The model under review builds one solid part; all positions refer to its coordinate system, in mm. Face numbers are marked on the shaded views. A direction names the side the tool comes from. Give positions to 0.01 mm unless a question says otherwise; leave off trailing zeros. Order: outer loops, then holes, each group sorted by start corner. A loop starts at its lowest first (then second) coordinate and runs counter-clockwise, first axis right, second up. Notation, with made-up numbers: (-5, 64) - (13, 64) arc R18 ccw to (13, 89) - close; hole circle Ø8 at (17.25, 0.5). An arc over 180 degrees is marked (long way). Write item = value, one per line. Start each with the question number.
1. We need section A-A, the plane y = 11. Give the boundary of the cut face in (x, z) (3 decimals).
2. We need section D-D, the plane z = 30. Give the boundary of the cut face in (x, y) (3 decimals), and give its area (3 significant figures).
3. We need section B-B, the plane z = 16.5. Give the boundary of the cut face in (x, y), and give its area (3 significant figures).
4. Wall thickness on probe 1 along X at (y, z) = (7.75, 17.5) (3 decimals); probe 2 along Y at (x, z) = (-45.5, 17); probe 3 along Y at (x, z) = (-27, 2): over which ranges is each line inside the solid? List them lowest first.
5. For P1, Ø4, axis at y = -7, z = 26, coming from the +X side; P2, Ø4.5, axis at y = 1, z = 32.5, coming from the -X side; P3, Ø5.5, axis at y = 0, z = 30, coming from the -X side; P4, Ø3, axis at x = -7, y = 0, coming from the +Z side, all flat-tipped, find the tip position at first contact; note any pin that passes through.
6. Mouldability with a two-part tool opening along Y and no side actions: class the marked faces 1, 2 and 3 as pulls with the +Y half, pulls with the -Y half, needs draft (parallel to the pull), parting line crosses it, or undercut.
7. Machinability: for the marked faces 4, 5 and 6, which of the approach directions +Z, -Z, +X, -X, +Y, -Y give a long, thin tool a straight path to every point of the face, cutting with its end or side? Answer none if there is none.
8. We need section C-C, the plane x = -27. Give the boundary of the cut face in (y, z).
from build123d import *

# Parameters (mm, degrees)
SKETCH1_R               = 1.575
BOSS_EXTRUDE1_DEPTH     = 12.5
SKETCH2_W               = 13.385271969
SKETCH2_H               = 10
CUT_EXTRUDE1_DEPTH      = 36
SKETCH3_R               = 1.75
CUT_EXTRUDE2_DEPTH      = 25
SKETCH4_R               = 4
CUT_EXTRUDE3_DEPTH      = 4
FILLET1_R               = 2
SKETCH5_R               = 2
CUT_EXTRUDE4_DEPTH      = 10
SKETCH7_R               = 3.575
CUT_EXTRUDE5_DEPTH      = 3.5
SKETCH8_R               = 10
CUT_EXTRUDE6_DEPTH      = 5
CUT_EXTRUDE6_DEPTH_BACK = 5
CUT_EXTRUDE7_DEPTH      = 3


with BuildPart() as part:
    # Sketch1 → Boss-Extrude1 (new body, symmetric)
    with BuildSketch(Plane(origin=(0, 0, 0), x_dir=(1, 0, 0), z_dir=(0, 1, 0))):
        Polygon((0, 0), (-43.5, 0), (-56.885271969, -10.457720596), (-56.885271969, -21.057720596), (-48.596177418, -32.057720596), (-43.5, -35), (-37, -35), (-37, -20), (0, -20), align=None)
        with Locations((-48.5, -17.5)):
            Circle(SKETCH1_R, mode=Mode.SUBTRACT)
    extrude(amount=BOSS_EXTRUDE1_DEPTH, both=True)

    # Sketch2 → Cut-Extrude1 (cut, through all)
    with BuildSketch(Plane.XY.offset(35)):
        with Locations((-50.192635985, 0)):
            Rectangle(SKETCH2_W, SKETCH2_H)
    extrude(amount=-CUT_EXTRUDE1_DEPTH, mode=Mode.SUBTRACT)

    # Sketch3 → Cut-Extrude2 (cut)
    with BuildSketch(Plane.XY.offset(20)):
        with Locations((-27, 0)):
            Circle(SKETCH3_R)
        with Locations((-7, 0)):
            Circle(SKETCH3_R)
    extrude(amount=-CUT_EXTRUDE2_DEPTH, mode=Mode.SUBTRACT)

    # Sketch4 → Cut-Extrude3 (cut)
    with BuildSketch(Plane(origin=(0, 0, 0), x_dir=(-1, 0, 0), z_dir=(0, 0, -1))):
        with Locations((7, 0)):
            Circle(SKETCH4_R)
        with Locations((27, 0)):
            Circle(SKETCH4_R)
    extrude(amount=-CUT_EXTRUDE3_DEPTH, mode=Mode.SUBTRACT)

    # Fillet1
    fillet1_edges = [part.edges().sort_by_distance(p)[0] for p in [
        (-56.885271969, 8.75, 21.057720596),
        (-56.885271969, 8.75, 10.457720596),
        (0, 0, 0),
        (-56.885271969, -8.75, 21.057720596),
        (-56.885271969, -8.75, 10.457720596),
    ]]
    fillet(fillet1_edges, radius=FILLET1_R)

    # Sketch5 → Cut-Extrude4 (cut)
    with BuildSketch(Plane.ZY.offset(43.5)):
        with Locations((30, 0)):
            Circle(SKETCH5_R)
    extrude(amount=-CUT_EXTRUDE4_DEPTH, mode=Mode.SUBTRACT)

    # Sketch7 → Cut-Extrude5 (cut)
    with BuildSketch(Plane.ZY.offset(43.5)):
        with Locations((30, 0)):
            Circle(SKETCH7_R)
    extrude(amount=-CUT_EXTRUDE5_DEPTH, mode=Mode.SUBTRACT)

    # Sketch8 → Cut-Extrude6 (cut, two sides)
    with BuildSketch(Plane(origin=(0, 0, 0), x_dir=(1, 0, 0), z_dir=(0, 1, 0))) as cut_extrude6_sk:
        with Locations((-48.5, -17.5)):
            Circle(SKETCH8_R)
    extrude(amount=CUT_EXTRUDE6_DEPTH, mode=Mode.SUBTRACT)
    extrude(cut_extrude6_sk.sketch, amount=-CUT_EXTRUDE6_DEPTH_BACK, mode=Mode.SUBTRACT)

    # Sketch9 → Cut-Extrude7 (cut)
    with BuildSketch(Plane.XZ.offset(12.5)):
        Polygon((-46.800589834, 14.481390206), (-45.036102151, 17.462427479), (-46.735512318, 20.481037272), (-50.199410166, 20.518609794), (-51.963897849, 17.537572521), (-50.264487682, 14.518962728), align=None)
    extrude(amount=-CUT_EXTRUDE7_DEPTH, mode=Mode.SUBTRACT)


solid = part.part
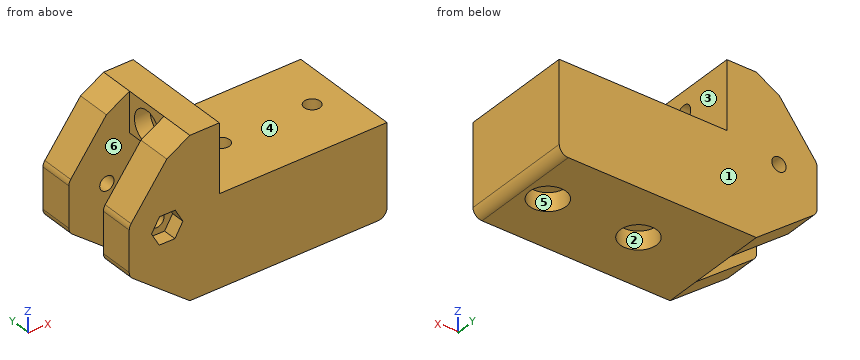
Model answer:
q1.outline = (-56.885, 11.433) arc R2 ccw to (-56.117, 9.857) - (-43.5, 0) - (-2, 0) arc R2 ccw to (0, 2) - (0, 20) - (-37, 20) - (-37, 35) - (-43.5, 35) - (-48.596, 32.058) - (-56.483, 21.592) arc R2 ccw to (-56.885, 20.389) - close; hole circle Ø3.15 at (-48.5, 17.5)
q2.outline = (-50.147, -12.5) - (-37, -12.5) - (-37, -2) - (-40, -2) - (-40, -3.575) - (-43.5, -3.575) - (-43.5, -5) - (-50.147, -5) - close; (-50.147, 5) - (-43.5, 5) - (-43.5, 3.575) - (-40, 3.575) - (-40, 2) - (-37, 2) - (-37, 12.5) - (-50.147, 12.5) - close
q2.area = 225 mm2
q3.outline = (-56.89, -12.5) - (-51.38, -12.5) - (-51.38, -9.5) - (-49.72, -9.5) - (-49.72, -5) - (-56.89, -5) - close; (-56.89, 5) - (-49.72, 5) - (-49.72, 12.5) - (-56.89, 12.5) - close; (-47.28, -9.5) - (-45.61, -9.5) - (-45.61, -12.5) - (0, -12.5) - (0, 12.5) - (-47.28, 12.5) - (-47.28, 5) - (-38.55, 5) - (-38.55, -5) - (-47.28, -5) - close; hole circle Ø3.5 at (-27, 0); hole circle Ø3.5 at (-7, 0)
q3.area = 1,170 mm2
q4.probe_1 = -56.885 to -50.075, -46.925 to 0
q4.probe_2 = -9.5 to -5, 5 to 12.5
q4.probe_3 = -12.5 to -4, 4 to 12.5
q5.P1 = -37
q5.P2 = -43.5
q5.P3 = -40
q5.P4 = through
q6.face_1 = pulls with the +Y half
q6.face_2 = undercut
q6.face_3 = needs draft
q7.face_4 = +Z, +X, +Y, -Y
q7.face_5 = -Z
q7.face_6 = -X
q8.outline = (-12.5, 0) - (-4, 0) - (-4, 4) - (-1.75, 4) - (-1.75, 20) - (-12.5, 20) - close; (1.75, 4) - (4, 4) - (4, 0) - (12.5, 0) - (12.5, 20) - (1.75, 20) - close
